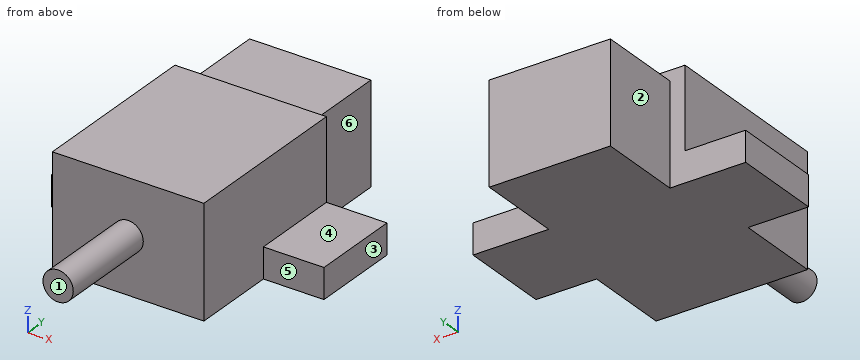
```python
from build123d import *

# Parameters (mm, degrees)
F0_W     = 12
F0_H     = 26
F1_DEPTH = 10
F2_W     = 15
F2_H     = 17.5
F3_DEPTH = 11
F4_W     = 9
F4_H     = 3
F5_DEPTH = 6
F6_W     = 9
F6_H     = 3
F7_DEPTH = 6
F8_R     = 1.5
F9_DEPTH = 10


# Not quite as in the source:
# - a feature names something its author has since deleted; it is built from what else it names


with BuildPart() as f1:
    # F0 (on Top) → F1 (new body)
    with BuildSketch(Plane.XY):
        with Locations((0, 13)):
            Rectangle(F0_W, F0_H)
    extrude(amount=F1_DEPTH)

    # F2 (on Top) → F3 (join)
    with BuildSketch(Plane.XY):
        with Locations((0, 8.75)):
            Rectangle(F2_W, F2_H)
    extrude(amount=F3_DEPTH)

    # F4 (on face) → F5 (join)
    with BuildSketch(Plane.YZ.offset(7.5)):
        with Locations((13, 1.5)):
            Rectangle(F4_W, F4_H)
    extrude(amount=F5_DEPTH)

    # F6 (on face) → F7 (join)
    with BuildSketch(Plane(origin=(-7.5, 0, 0), x_dir=(0, -1, 0), z_dir=(-1, 0, 0))):
        with Locations((-13, 1.5)):
            Rectangle(F6_W, F6_H)
    extrude(amount=F7_DEPTH)

    # F8 (on face) → F9 (join)
    with BuildSketch(Plane.XZ):
        with Locations((0, 5.5)):
            Circle(F8_R)
    extrude(amount=F9_DEPTH)


solid = f1.part
```
Check sheet for the modelled part. Datum: model origin and axes. Units: mm. Face numbers are marked on the shaded views. A direction names the side the tool comes from. Round coordinates to 2 decimals unless told otherwise and drop trailing zeros. Write each loop counter-clockwise with the first axis right and the second up, starting at its lowest first coordinate (ties: lowest second). Pieces come first, ordered by that corner, then holes. Notation, with made-up numbers: M -24,-9.5 L 15,-9.5 A13 cw 15,13.5 Z; hole C -18,69.25 d10. An arc over 180 degrees is marked long. Write item = value, one per line. Start each with the question number.
1. Section check B-B, the plane z = 5.5. Record the cut outline in (x, y).
2. Release check for a two-part mould opening along X. For the marked faces 1, 2 and 3 record: pulls with the +X half, pulls with the -X half, needs draft (parallel to the pull), parting line crosses it, or undercut.
3. Tool access check on the marked faces 4, 5 and 6. Record the directions out of +Z, -Z, +X, -X, +Y, -Y that give a thin tool (end or side, any length) a straight path to the whole face; none if there is none.
4. Section check C-C, the plane y = 14. Record the cut outline in (x, z).
5. Section check D-D, the plane z = 8. Record the cut outline in (x, y).
6. Scan lines: line 1 (X direction, y = 6.5, z = 4); line 2 (Y direction, x = 12, z = 2.5); line 3 (X direction, y = 20.5, z = 8.25). Record each from-to range of solid material in increasing order. Write a range as [from, to].
7. Gauge pin test, flat ends, axial feed: pin 1 (5.5 mm diameter, centred on y = 11.5, z = 7, fed in from +X); pin 2 (3.5 mm diameter, centred on y = 11, z = 6.5, fed in from -X); pin 3 (1.5 mm diameter, centred on x = -0.5, z = 9, fed in from -Y). Record the tip position at first contact, or that the pin passes through.
8. Section check A-A, the plane x = 0. Record the cut outline in (y, z).
Results found:
q1.outline = M -7.5,0 L -1.5,0 L -1.5,-10 L 1.5,-10 L 1.5,0 L 7.5,0 L 7.5,17.5 L 6,17.5 L 6,26 L -6,26 L -6,17.5 L -7.5,17.5 Z
q2.face_1 = needs draft
q2.face_2 = pulls with the -X half
q2.face_3 = pulls with the +X half
q3.face_4 = +Z, +X, +Y, -Y
q3.face_5 = +Z, -Z, +X, -Y
q3.face_6 = +Z, -Z, +X, +Y
q4.outline = M -13.5,0 L 13.5,0 L 13.5,3 L 7.5,3 L 7.5,11 L -7.5,11 L -7.5,3 L -13.5,3 Z
q5.outline = M -7.5,0 L 7.5,0 L 7.5,17.5 L 6,17.5 L 6,26 L -6,26 L -6,17.5 L -7.5,17.5 Z
q6.line_1 = [-7.5, 7.5]
q6.line_2 = [8.5, 17.5]
q6.line_3 = [-6, 6]
q7.pin_1 = 7.5
q7.pin_2 = -7.5
q7.pin_3 = 0
q8.outline = M -10,4 L 0,4 L 0,0 L 26,0 L 26,10 L 17.5,10 L 17.5,11 L 0,11 L 0,7 L -10,7 Z
